The drawing under review shows one solid part. Ordinate dimensions are in mm from its lowest x, y, z. Coordinates: 2 decimals unless noted, no trailing zeros. Write each loop counter-clockwise with the first axis right and the second up, starting at its lowest first coordinate (ties: lowest second). Pieces come first, ordered by that corner, then holes. Notation, with made-up numbers: (64, -40) - (108, -40) arc R25 cw to (108, -16) - close; hole circle Ø2 at (12, -16.5). An arc over 180 degrees is marked (long way). Answer as CSV lines item,"result". Start each with the question number.
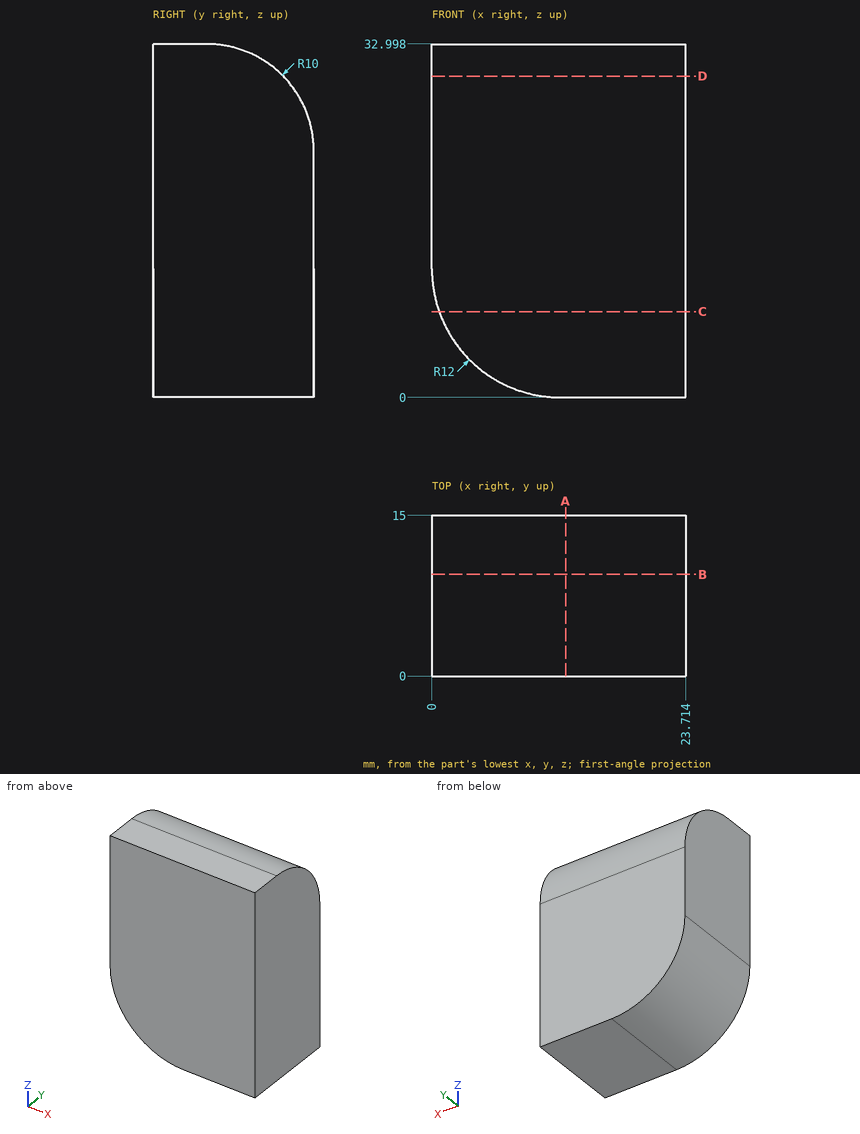
(1) Wall thickness on line 1 (Z direction, x = 13.25, y = 5.25) (1 decimal); line 2 (X direction, y = 5.75, z = 2.5) (1 decimal); line 3 (Z direction, x = 22.5, y = 7.25): over which ranges is each line inside the solid? List them lowest first.
(2) Add section C-C on z = 8. Give the boundary of the cut face in (x, y), then the cut area to 3 significant figures.
(3) Add section B-B on y = 9.5. Give the boundary of the cut face in (x, z).
(4) Add section D-D on z = 30. Give the boundary of the cut face in (x, y), then the cut area to 3 significant figures.
(5) Add section A-A on x = 12.5. Give the boundary of the cut face in (y, z).
(6) For pin 1 (8 mm diameter, centred on x = 14, z = 28.5, fed in from +Y); pin 2 (1.5 mm diameter, centred on x = 16.5, y = 9, fed in from +Z) (1 decimal), all flat-tipped, find the tip position at first contact; note any pin that passes through.
Reported:
1,line 1,"0 to 33"
1,line 2,"4.7 to 23.7"
1,line 3,"0 to 32.74"
2,outline,"(0.69, 0) - (23.71, 0) - (23.71, 15) - (0.69, 15) - close"
2,area,"345 mm²"
3,outline,"(0, 12) arc R12 ccw to (12, 0) - (23.71, 0) - (23.71, 31.93) - (0, 31.93) - close"
4,outline,"(0, 0) - (23.71, 0) - (23.71, 12.14) - (0, 12.14) - close"
4,area,"288 mm²"
5,outline,"(0, 0) - (15, 0) - (15, 23) arc R10 ccw to (5, 33) - (0, 33) - close"
6,pin 1,"y = 14.89"
6,pin 2,"z = 32.5"
